CAD build for the part. Positions are in the model's coordinates, mm. Round coordinates to 2 decimals unless told otherwise and drop trailing zeros. Loops run counter-clockwise (first coordinate to the right, second up) from the corner with the lowest first, then second, coordinate; pieces in that order, holes last.
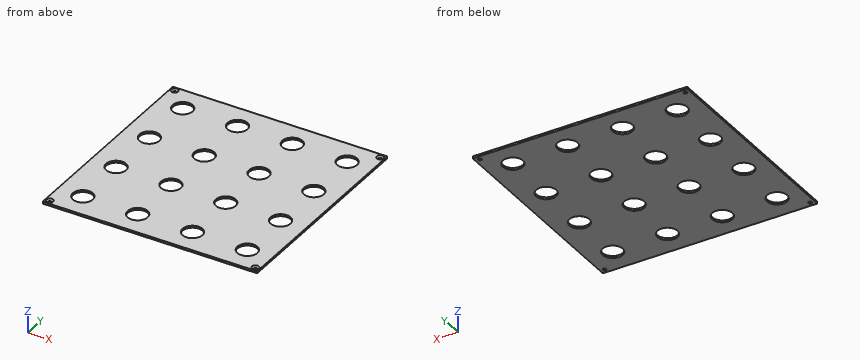
```python
from build123d import *

# Parameters (mm, degrees)
PAD_DEPTH        = 1
POCKET_DEPTH     = 0.001
HOLE_D           = 1.75
HOLE_CSINK_D     = 3.3
HOLE_CSINK_ANGLE = 90
SKETCH005_R      = 4.85
HOLE003_DEPTH    = 1.001


with BuildPart() as part:
    # Sketch → Pad (new body)
    with BuildSketch(Plane.XY):
        with BuildLine():
            Line((-51.8, 52.175), (51.8, 52.175))
            ThreePointArc((52.175, 51.8), (52.065165, 52.065165), (51.8, 52.175))
            Line((52.175, 51.8), (52.175, -51.8))
            ThreePointArc((51.8, -52.175), (52.065165, -52.065165), (52.175, -51.8))
            Line((51.8, -52.175), (-51.8, -52.175))
            ThreePointArc((-52.175, -51.8), (-52.065165, -52.065165), (-51.8, -52.175))
            Line((-52.175, -51.8), (-52.175, 51.8))
            ThreePointArc((-51.8, 52.175), (-52.065165, 52.065165), (-52.175, 51.8))
        make_face()
    extrude(amount=-PAD_DEPTH)

    # Sketch002 → Pocket (cut, through all)
    with BuildSketch(Plane.XY.offset(-4.8)):
        with BuildLine():
            Line((-45, 50.175), (45, 50.175))
            ThreePointArc((45, 50.175), (45.353553, 50.321447), (45.5, 50.675))
            ThreePointArc((45.5, 50.675), (45.353553, 51.028553), (45, 51.175))
            Line((-45, 51.175), (45, 51.175))
            ThreePointArc((-45, 51.175), (-45.353553, 51.028553), (-45.5, 50.675))
            ThreePointArc((-45.5, 50.675), (-45.353553, 50.321447), (-45, 50.175))
        make_face()
        with BuildLine():
            Line((-45, -51.175), (45, -51.175))
            ThreePointArc((45, -51.175), (45.353553, -51.028553), (45.5, -50.675))
            ThreePointArc((45.5, -50.675), (45.353553, -50.321447), (45, -50.175))
            Line((-45, -50.175), (45, -50.175))
            ThreePointArc((-45, -50.175), (-45.353553, -50.321447), (-45.5, -50.675))
            ThreePointArc((-45.5, -50.675), (-45.353553, -51.028553), (-45, -51.175))
        make_face()
        with BuildLine():
            Line((51.175, -45), (51.175, 45))
            ThreePointArc((51.175, 45), (51.028553, 45.353553), (50.675, 45.5))
            ThreePointArc((50.675, 45.5), (50.321447, 45.353553), (50.175, 45))
            Line((50.175, -45), (50.175, 45))
            ThreePointArc((50.175, -45), (50.321447, -45.353553), (50.675, -45.5))
            ThreePointArc((50.675, -45.5), (51.028553, -45.353553), (51.175, -45))
        make_face()
        with BuildLine():
            Line((-50.175, -45), (-50.175, 45))
            ThreePointArc((-50.175, 45), (-50.321447, 45.353553), (-50.675, 45.5))
            ThreePointArc((-50.675, 45.5), (-51.028553, 45.353553), (-51.175, 45))
            Line((-51.175, -45), (-51.175, 45))
            ThreePointArc((-51.175, -45), (-51.028553, -45.353553), (-50.675, -45.5))
            ThreePointArc((-50.675, -45.5), (-50.321447, -45.353553), (-50.175, -45))
        make_face()
    extrude(amount=-POCKET_DEPTH, mode=Mode.SUBTRACT)

    # Hole (through all)
    with Locations(Plane.XY):
        with Locations((-50, 50), (50, 50), (50, -50), (-50, -50)):
            CounterSinkHole(HOLE_D / 2, HOLE_CSINK_D / 2, counter_sink_angle=HOLE_CSINK_ANGLE)

    # Sketch005 → Hole003 (cut, through all)
    with BuildSketch(Plane.XY):
        with Locations((-40.005, 40.005)):
            Circle(SKETCH005_R)
        with Locations((-13.335, 40.005)):
            Circle(SKETCH005_R)
        with Locations((13.335, 40.005)):
            Circle(SKETCH005_R)
        with Locations((40.005, 40.005)):
            Circle(SKETCH005_R)
        with Locations((-40.005, 13.335)):
            Circle(SKETCH005_R)
        with Locations((-13.335, 13.335)):
            Circle(SKETCH005_R)
        with Locations((13.335, 13.335)):
            Circle(SKETCH005_R)
        with Locations((40.005, 13.335)):
            Circle(SKETCH005_R)
        with Locations((-40.005, -13.335)):
            Circle(SKETCH005_R)
        with Locations((-13.335, -13.335)):
            Circle(SKETCH005_R)
        with Locations((13.335, -13.335)):
            Circle(SKETCH005_R)
        with Locations((40.005, -13.335)):
            Circle(SKETCH005_R)
        with Locations((-40.005, -40.005)):
            Circle(SKETCH005_R)
        with Locations((-13.335, -40.005)):
            Circle(SKETCH005_R)
        with Locations((13.335, -40.005)):
            Circle(SKETCH005_R)
        with Locations((40.005, -40.005)):
            Circle(SKETCH005_R)
    extrude(amount=-HOLE003_DEPTH, mode=Mode.SUBTRACT)


solid = part.part
```
Item 1: Flat gauge pins, fed straight in: P1, Ø12, axis at x = 41.5, y = 11, coming from the -Z side; P2, Ø3, axis at x = -50, y = -50, coming from the +Z side. Where does each tip first touch, or does it go through?
Answers follow:
P1: stops at z = -1
P2: stops at z = -0.15
Item 2: Probe line 1 (Y direction, x = 50, z = -0.85) (3 decimals); line 2 (X direction, y = -12.5, z = -0.3) (3 decimals); line 3 (Y direction, x = -17, z = -0.65) (3 decimals). List the from-to ranges inside material, lowest first.
Answers follow:
line 1: y = -52.175 to -50.875, -49.125 to 49.125, 50.875 to 52.175
line 2: x = -52.175 to -44.783, -35.227 to -18.113, -8.557 to 8.557, 18.113 to 35.227, 44.783 to 52.175
line 3: y = -52.175 to -43.182, -36.828 to -16.512, -10.158 to 10.158, 16.512 to 36.828, 43.182 to 52.175
Item 3: Cut at C-C, the plane y = 15. Give the cut face in (x, z) (3 decimals).
Answers follow:
outline: (-52.175, -1) - (-44.56, -1) - (-44.56, 0) - (-52.175, 0) - close; (-35.45, -1) - (-17.89, -1) - (-17.89, 0) - (-35.45, 0) - close; (-8.78, -1) - (8.78, -1) - (8.78, 0) - (-8.78, 0) - close; (17.89, -1) - (35.45, -1) - (35.45, 0) - (17.89, 0) - close; (44.56, -1) - (52.175, -1) - (52.175, 0) - (44.56, 0) - close
Item 4: Cut at B-B, the plane z = -0.5. State how many separate pieces and enclosed holes the cut face has, plus the area to 3 significant figures.
Answers follow:
separate pieces: 1
enclosed holes: 20
area: 9,690 mm2
Item 5: Cut at A-A, the plane y = -42. Give the cut face in (x, z) (3 decimals).
Answers follow:
outline: (-52.175, -1) - (-44.426, -1) - (-44.426, 0) - (-52.175, 0) - close; (-35.584, -1) - (-17.756, -1) - (-17.756, 0) - (-35.584, 0) - close; (-8.914, -1) - (8.914, -1) - (8.914, 0) - (-8.914, 0) - close; (17.756, -1) - (35.584, -1) - (35.584, 0) - (17.756, 0) - close; (44.426, -1) - (52.175, -1) - (52.175, 0) - (44.426, 0) - close
